```python
from build123d import *

# Parameters (mm, degrees)
SKETCH1_W           = 55
SKETCH1_H           = 70
BOSS_EXTRUDE1_DEPTH = 110
SKETCH2_R           = 14
CUT_EXTRUDE1_DEPTH  = 108
SKETCH3_W           = 5
SKETCH3_H           = 32
CUT_EXTRUDE2_DEPTH  = 18
SKETCH4_R           = 17
CUT_EXTRUDE3_DEPTH  = 13.5
CUT_EXTRUDE5_REACH  = 137.341
SKETCH5_R           = 19
CUT_EXTRUDE7_REACH  = 143.51
CUT_EXTRUDE8_REACH  = 143.51


with BuildPart() as part:
    # Sketch1 → Boss-Extrude1 (new body)
    with BuildSketch(Plane(origin=(0, 0, 0), x_dir=(1, 0, 0), z_dir=(0, 1, 0))):
        with Locations((27.5, 35)):
            Rectangle(SKETCH1_W, SKETCH1_H)
    extrude(amount=BOSS_EXTRUDE1_DEPTH)

    # Sketch2 → Cut-Extrude1 (cut)
    with BuildSketch(Plane(origin=(0, 110, 0), x_dir=(1, 0, 0), z_dir=(0, 1, 0))):
        with Locations(Location((39, 16, 0), (0, 0, 270))):
            Circle(SKETCH2_R)
    extrude(amount=-CUT_EXTRUDE1_DEPTH, mode=Mode.SUBTRACT)

    # Sketch3 → Cut-Extrude2 (cut)
    with BuildSketch(Plane(origin=(0, 110, 0), x_dir=(1, 0, 0), z_dir=(0, 1, 0))):
        with Locations((52.5, 16)):
            Rectangle(SKETCH3_W, SKETCH3_H)
        Polygon((0, 0), (18, 0), (18, 8), (31.332818552, 8), (31.332818552, 24), (18, 24), (18, 32), (0, 32), align=None)
    extrude(amount=-CUT_EXTRUDE2_DEPTH, mode=Mode.SUBTRACT)

    # Sketch4 → Cut-Extrude3 (cut)
    with BuildSketch(Plane(origin=(0, 0, -70), x_dir=(-1, 0, 0), z_dir=(0, 0, -1))):
        with Locations((-16, 110)):
            Circle(SKETCH4_R)
    extrude(amount=-CUT_EXTRUDE3_DEPTH, mode=Mode.SUBTRACT)

    # Cut-Extrude5: up to this face of the body (flat: up to its plane)
    cut_extrude5_end = Plane(part.part.faces().sort_by_distance((22.755437353, 101, -24))[0])
    # Sketch5 → Cut-Extrude5 (cut, up to the picked face)
    with BuildSketch(Plane(origin=(0, 0, -56.5), x_dir=(-1, 0, 0), z_dir=(0, 0, -1)), mode=Mode.PRIVATE) as cut_extrude5_sk1:
        with Locations((-16.5, 110)):
            Circle(SKETCH5_R)
    cut_extrude5_tool1 = split(extrude(cut_extrude5_sk1.sketch, amount=-CUT_EXTRUDE5_REACH, mode=Mode.PRIVATE), bisect_by=cut_extrude5_end, keep=Keep.BOTH, mode=Mode.PRIVATE)
    add(cut_extrude5_tool1.solids().sort_by(Axis((16.5, 110, -56.5), (0, 0, 1)))[0], mode=Mode.SUBTRACT)

    # Sketch8 → Cut-Extrude7 (cut, up to next)
    with BuildSketch(Plane(origin=(55, 0, 0), x_dir=(0, 0, -1), z_dir=(1, 0, 0)), mode=Mode.PRIVATE) as cut_extrude7_sk1:
        Polygon((70, 0), (70, 80), (35, 0), align=None)
    cut_extrude7_tool1 = extrude(cut_extrude7_sk1.sketch, amount=-CUT_EXTRUDE7_REACH, mode=Mode.PRIVATE) & part.part
    add(cut_extrude7_tool1.solids().sort_by_distance((55, 26.666667, -58.333333))[0], mode=Mode.SUBTRACT)

    # Cut-Extrude8: up to this plane
    cut_extrude8_end = Plane(origin=(-0.001, 80, -70), z_dir=(0, 0.40081883401970747, 0.9161573349021893))
    # Sketch9 → Cut-Extrude8 (cut, up to the surface)
    with BuildSketch(Plane.XY, mode=Mode.PRIVATE) as cut_extrude8_sk1:
        Polygon((0, 0), (25, 0), (0, 80), align=None)
    cut_extrude8_tool1 = split(extrude(cut_extrude8_sk1.sketch, amount=-CUT_EXTRUDE8_REACH, mode=Mode.PRIVATE), bisect_by=cut_extrude8_end, keep=Keep.BOTH, mode=Mode.PRIVATE)
    add(cut_extrude8_tool1.solids().sort_by_distance((8.333333, 26.666667, 0))[0], mode=Mode.SUBTRACT)


solid = part.part
```
Work out the finished part from the listing and answer in its coordinate system (mm). A direction names the side the tool comes from. Coordinates: 2 decimals unless noted, no trailing zeros. Write each loop counter-clockwise with the first axis right and the second up, starting at its lowest first coordinate (ties: lowest second). Pieces come first, ordered by that corner, then holes.
Q1. Determine the mould class of faces 5 (the face through (50, 101, -28)), 6 (the face through (23, 101, -8)), 7 (the face through (23, 94, -56.5)), 8 (the face through (39, 2, -16)) for opening direction X: released by +X, released by -X, zero draft, split by the parting line, or undercut.
Q2. Find the intervals of material crossed by line 1 (Z direction, x = 39, y = 82); line 2 (X direction, y = 81, z = -16); line 3 (X direction, y = 99.5, z = -53.5), in increasing order.
Q3. A cutting plane is placed at B-B, the plane x = 39. Give the vertices of the cut face in (y, z), then the cut area to 3 significant figures.
Q4. A cutting plane is placed at A-A, the plane z = -16. Give the vertices of the cut face in (x, y), then the cut area to 3 significant figures.
Q5. Each of these flat-tipped pins is pushed along its axis until it touches: pin 1 Ø8 at (y, z) = (97.5, -3.5) entering from +X; pin 2 Ø2.5 at (y, z) = (104, -4.5) entering from -X; pin 3 Ø4 at (x, z) = (8, -27) entering from +Y. Where does it stop, or does it pass through?
Q6. A cutting plane is placed at C-C, the plane y = 15.5. Give the vertices of the cut face in (x, z), then the cut area to 3 significant figures.
Q7. Which of the six approach directions +Z, -Z, +X, -X, +Y, -Y give full straight-line access (tool end or side, diameter ignored) to faces 1 (the face through (3, 94, -32)), 2 (the face through (50, 101, -4)), 3 (the face through (48.46, 56.76, -26.32)), 4 (the face through (26, 93, -24))?
Q8. A cutting plane is placed at D-D, the plane y = 27.5. Give the vertices of the cut face in (x, z), then the cut area to 3 significant figures.
Findings below:
1. face 5: released by +X
1. face 6: zero draft
1. face 7: undercut
1. face 8: undercut
2. line 1: z = -70 to -30, -2 to 0
2. line 2: x = 0 to 25, 53 to 55
2. line 3: x = 0 to 0.66, 32.34 to 55
3. outline: (0, -35) - (80, -70) - (110, -70) - (110, -30) - (2, -30) - (2, -2) - (110, -2) - (110, 0) - (0, 0) - close
3. area: 3,280 mm2
4. outline: (0, 80) - (25, 0) - (55, 0) - (55, 92) - (53, 92) - (53, 2) - (25, 2) - (25, 92) - (0, 92) - close
4. area: 1,540 mm2
5. pin 1: stops at x = 50
5. pin 2: stops at x = 18
5. pin 3: stops at y = 92
6. outline: (20.16, -41.78) - (55, -41.78) - (55, 0) - (20.16, 0) - close; hole circle Ø28 at (39, -16)
6. area: 840 mm2
7. face 1: +Z, -X, +Y
7. face 2: +Z, +X, +Y
7. face 3: +Y
7. face 4: +X, -X, +Y
8. outline: (16.41, -47.03) - (55, -47.03) - (55, 0) - (16.41, 0) - close; hole circle Ø28 at (39, -16)
8. area: 1,200 mm2
